Study the drawing (mm; zero at the part's minimum x, y, z) and answer. A direction names the side the tool comes from. Coordinates: 2 decimals unless noted, no trailing zeros. Order: outer loops, then holes, each group sorted by start corner. A loop starts at its lowest first (then second) coordinate and runs counter-clockwise, first axis right, second up. Notation, with made-up numbers: (-3, 58) -> (45, 58) arc R10 ccw to (45, 62) -> close; hole circle Ø4 at (72.5, 19.5). An arc over 180 degrees is marked (long way). Answer as CSV lines item,"result". Start each with the question number.
Item 1: Section C-C (x = 43.5) is taken. Write down the section's boundary in (y, z).
Item 2: Section B-B (y = 32) is taken. Write down the section's boundary in (x, z) (1 decimal).
Item 3: Straight lines are drawn through the part: L1, parallel to X at y = 40, z = 13 (1 decimal); L2, parallel to X at y = 38.5, z = 27.5 (1 decimal); L3, parallel to Y at x = 50, z = 16.5 (1 decimal). For each, find the intervals that lie inside material, in ascending order.
Item 4: Section A-A (x = 54.5) is taken. Write down the section's boundary in (y, z).
Item 5: Section D-D (z = 38) is taken. Write down the section's boundary in (x, y).
Item 6: Which of the six approach directions +Z, -Z, +X, -X, +Y, -Y give full straight-line access (tool end or side, diameter ignored) to the marked faces 1 and 2?
Item 7: Each of these flat-tipped pins is pushed along its axis until it touches: pin 1 Ø8 at (x, y) = (13.5, 83) entering from +Z; pin 2 Ø12 at (x, y) = (56.2, 33.97) entering from -Z; pin 3 Ø1 at (x, y) = (61, 16) entering from +Z; pin 4 Ø14 at (x, z) = (55, 50) entering from -Y. Where does it stop, or does it pass through?
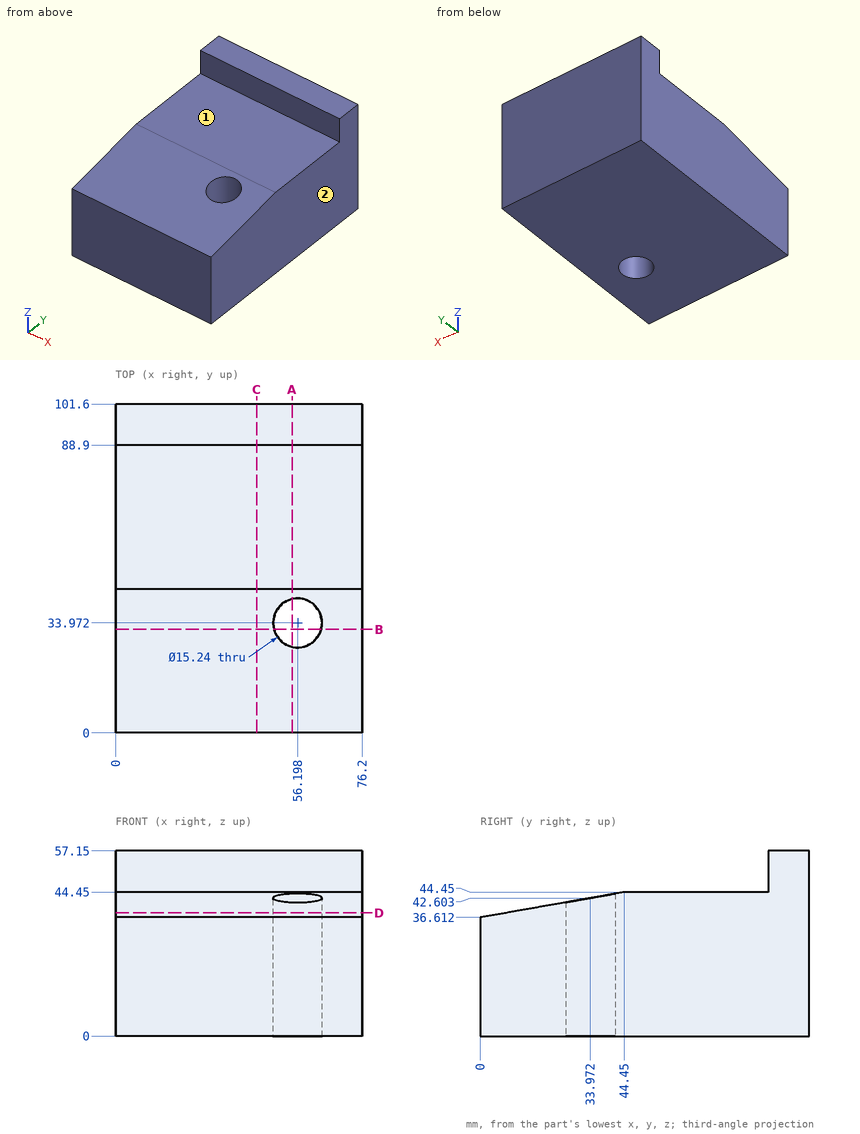
Checked values:
1,outline,"(0, 0) -> (101.6, 0) -> (101.6, 57.15) -> (88.9, 57.15) -> (88.9, 44.45) -> (44.45, 44.45) -> (0, 36.61) -> close"
2,outline,"(0, 0) -> (48.8, 0) -> (48.8, 42.3) -> (0, 42.3) -> close; (63.6, 0) -> (76.2, 0) -> (76.2, 42.3) -> (63.6, 42.3) -> close"
3,L1,"x = 0 to 51.5, 60.9 to 76.2"
3,L2,"x = 0 to 50.1, 62.3 to 76.2"
3,L3,"y = 0 to 29.5, 38.4 to 101.6"
4,outline,"(0, 0) -> (26.54, 0) -> (26.54, 41.29) -> (0, 36.61) -> close; (41.4, 0) -> (101.6, 0) -> (101.6, 57.15) -> (88.9, 57.15) -> (88.9, 44.45) -> (44.45, 44.45) -> (41.4, 43.91) -> close"
5,outline,"(0, 7.87) -> (76.2, 7.87) -> (76.2, 101.6) -> (0, 101.6) -> close; hole circle Ø15.24 at (56.2, 33.97)"
6,face 1,"+Z, +X, -X, -Y"
6,face 2,"+Z, -Z, +X, +Y, -Y"
7,pin 1,"stops at z = 44.45"
7,pin 2,"passes through"
7,pin 3,"stops at z = 39.52"
7,pin 4,"stops at y = 40.28"
